The figure shows three views and two pictorial views of one solid part (mm, origin at its lowest corner). Answer the questions. A direction names the side the tool comes from. Coordinates: 2 decimals unless noted, no trailing zeros. Loops run counter-clockwise (first coordinate to the right, second up) from the corner with the lowest first, then second, coordinate; pieces in that order, holes last. Notation, with made-up numbers: (66, 87.25) - (76, 87.25) arc R10 cw to (76, 105.25) - close; hole circle Ø11 at (37, 64.25). An arc over 180 degrees is marked (long way). Return JSON: item names as keys, results as strings. Group by question number.
1. Section A-A (x = 7.5) is taken. Write down the section's boundary in (y, z) (3 decimals).
2. Section D-D (y = 3) is taken. Write down the section's boundary in (x, z) (3 decimals), and give its area (3 significant figures).
3. Each of these flat-tipped pins is pushed along its axis until it touches: P1, Ø4, axis at x = 2.5, y = 4, coming from the -Z side; P2, Ø1, axis at y = 11, z = 13.5, coming from the +X side; P3, Ø1.5, axis at y = 4.5, z = 3, coming from the -X side; P4, Ø2, axis at x = 7.5, y = 5, coming from the +Z side. Where does it stop, or does it pass through?
4. Section B-B (z = 7.5) is taken. Write down the section's boundary in (x, y) (3 decimals).
5. Section C-C (y = 26) is taken. Write down the section's boundary in (x, z), and give its area (3 significant figures).
6. Which of the six approach directions +Z, -Z, +X, -X, +Y, -Y give full straight-line access (tool end or side, diameter ignored) to the marked faces 1, 2 and 3?
7. Find the intervals of material crossed by line 1 along Z through (x, y) = (4, 28); line 2 along Z through (x, y) = (6.75, 2); line 3 along Y through (x, z) = (12.25, 8.5), in increasing order.
8. The mould has two halves that part along Z. Classify the marked faces 4, 5 and 6: pulls with the +Z half, pulls with the -Z half, needs draft (parallel to the pull), parting line crosses it, or undercut.
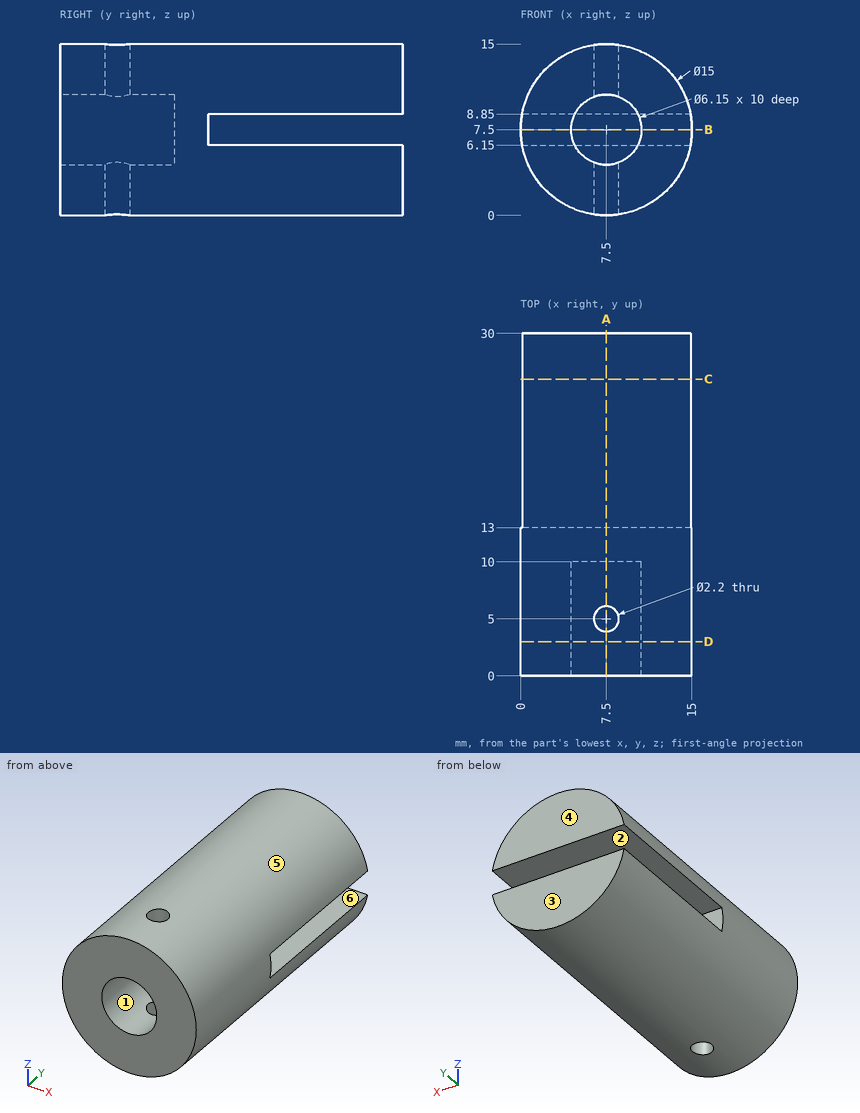
The answers:
{
 "1": {"outline": "(0, 0) - (3.9, 0) - (3.9, 4.425) - (0, 4.425) - close; (0, 10.575) - (3.9, 10.575) - (3.9, 15) - (0, 15) - close; (6.1, 0) - (30, 0) - (30, 6.15) - (13, 6.15) - (13, 8.85) - (30, 8.85) - (30, 15) - (6.1, 15) - (6.1, 10.575) - (10, 10.575) - (10, 4.425) - (6.1, 4.425) - close"},
 "2": {"outline": "circle Ø15 at (7.5, 7.5); hole circle Ø6.15 at (7.5, 7.5)", "area": "147 mm2"},
 "3": {"P1": "stops at z = 0.63", "P2": "stops at x = 12.6", "P3": "stops at x = 1", "P4": "passes through"},
 "4": {"outline": "(0, 0) - (4.425, 0) - (4.425, 10) - (10.575, 10) - (10.575, 0) - (15, 0) - (15, 13) - (0, 13) - close"},
 "5": {"outline": "(0.12, 6.15) arc R7.5 ccw to (14.88, 6.15) - close; (0.12, 8.85) - (14.88, 8.85) arc R7.5 ccw to start", "area": "136 mm2"},
 "6": {"face 1": "-Y", "face 2": "+X, -X, +Y", "face 3": "+Z, -Z, +X, -X, +Y"},
 "7": {"line 1": "z = 0.87 to 6.15, 8.85 to 14.13", "line 2": "z = 0.04 to 4.52, 10.48 to 14.96", "line 3": "y = 0 to 13"},
 "8": {"face 4": "needs draft", "face 5": "parting line crosses it", "face 6": "undercut"}
}
